from build123d import *

# Parameters (mm, degrees)
F1_DEPTH       = 6.35
F2_R           = 3.81
F3_DEPTH       = 6.35
F5_D           = 2.0574
F5_CSINK_D     = 4.2672
F5_CSINK_ANGLE = 82
F6_D           = 2.032
F6_CSINK_D     = 3.175
F6_CSINK_ANGLE = 82


with BuildPart() as f1:
    # F0 (on Top) → F1 (new body)
    with BuildSketch(Plane.XY):
        with BuildLine():
            ThreePointArc((-6.35, 12.7), (-4.4901280605, 8.2098719395), (0, 6.35))
            Line((0, 6.35), (0, 12.7))
            Line((0, 12.7), (0, 19.05))
            ThreePointArc((0, 19.05), (-4.4901280605, 17.1901280605), (-6.35, 12.7))
        make_face()
        with BuildLine():
            Line((0, 12.7), (0, 6.35))
            ThreePointArc((0, 6.35), (4.4901280605, 8.2098719395), (6.35, 12.7))
            ThreePointArc((6.35, 12.7), (4.4901280605, 17.1901280605), (0, 19.05))
            Line((0, 19.05), (0, 12.7))
        make_face()
        with BuildLine():
            ThreePointArc((6.35, 12.7), (4.4901280605, 8.2098719395), (0, 6.35))
            ThreePointArc((0, 6.35), (-4.4901280605, 8.2098719395), (-6.35, 12.7))
            Line((-6.35, 12.7), (-6.35, 0))
            ThreePointArc((-6.35, 0), (0, -6.35), (6.35, 0))
            Line((6.35, 0), (6.35, 12.7))
        make_face()
        with BuildLine():
            ThreePointArc((0, 19.05), (4.4901280605, 17.1901280605), (6.35, 12.7))
            Line((6.35, 12.7), (6.35, 32.3486101727))
            Line((6.35, 32.3486101727), (5.2643885857, 30.739125063))
            ThreePointArc((5.2643885857, 30.739125063), (2.9811444237, 28.6832827853), (0, 27.94))
            Line((0, 27.94), (0, 19.05))
        make_face()
        with BuildLine():
            Line((-6.35, 34.29), (-6.35, 12.7))
            ThreePointArc((-6.35, 12.7), (-4.4901280605, 17.1901280605), (0, 19.05))
            Line((0, 19.05), (0, 27.94))
            ThreePointArc((0, 27.94), (-4.4901280605, 29.7998719395), (-6.35, 34.29))
        make_face()
        with BuildLine():
            Line((6.35, 34.29), (6.35, 32.3486101727))
            Line((6.35, 32.3486101727), (27.9899881828, 64.4312120116))
            ThreePointArc((27.9899881828, 64.4312120116), (26.2764745341, 73.2464755344), (17.4612110113, 71.5329618857))
            Line((17.4612110113, 71.5329618857), (-5.2643885857, 37.840874937))
            ThreePointArc((-5.2643885857, 37.840874937), (-1.2116371206, 40.5233326149), (3.550874937, 39.5543885857))
            ThreePointArc((3.550874937, 39.5543885857), (5.6067172147, 37.2711444237), (6.35, 34.29))
        make_face()
        with BuildLine():
            Line((5.2643885857, 30.739125063), (6.35, 32.3486101727))
            Line((6.35, 32.3486101727), (6.35, 34.29))
            ThreePointArc((6.35, 34.29), (5.6067172147, 37.2711444237), (3.550874937, 39.5543885857))
            Line((3.550874937, 39.5543885857), (0, 34.29))
            Line((0, 34.29), (0, 27.94))
            ThreePointArc((0, 27.94), (2.9811444237, 28.6832827853), (5.2643885857, 30.739125063))
        make_face()
        with BuildLine():
            ThreePointArc((-5.2643885857, 37.840874937), (-6.0725352004, 36.146560325), (-6.35, 34.29))
            ThreePointArc((-6.35, 34.29), (-4.4901280605, 29.7998719395), (0, 27.94))
            Line((0, 27.94), (0, 34.29))
            Line((0, 34.29), (3.550874937, 39.5543885857))
            ThreePointArc((3.550874937, 39.5543885857), (-1.2116371206, 40.5233326149), (-5.2643885857, 37.840874937))
        make_face()
    extrude(amount=F1_DEPTH)

    # F2 (on face) → F3 (join)
    with BuildSketch(Plane.XY.offset(6.35)):
        with Locations((0, 12.7)):
            Circle(F2_R)
    extrude(amount=F3_DEPTH)

    # F5 (through all)
    with Locations(Plane.XY.offset(12.7)):
        with Locations((0, 12.7)):
            CounterSinkHole(F5_D / 2, F5_CSINK_D / 2, counter_sink_angle=F5_CSINK_ANGLE)

    # F6 (through all)
    with Locations(Plane(origin=(0, 0, 0), x_dir=(1, 0, 0), z_dir=(0, 0, -1))):
        with Locations((0, 0)):
            CounterSinkHole(F6_D / 2, F6_CSINK_D / 2, counter_sink_angle=F6_CSINK_ANGLE)


solid = f1.part
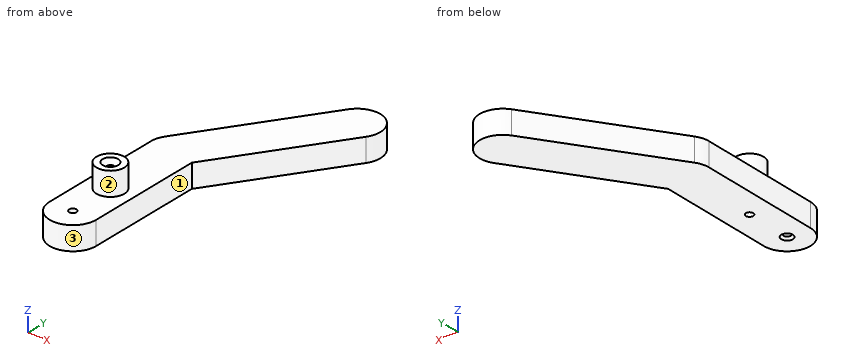
Geometry: final body of the model. Coordinates: model frame, mm. Face numbers are marked on the shaded views. A direction names the side the tool comes from. Give positions to 0.01 mm unless a question says otherwise; leave off trailing zeros. Loops run counter-clockwise (first coordinate to the right, second up) from the corner with the lowest first, then second, coordinate; pieces in that order, holes last. Notation, with made-up numbers: (2, 77) - (44, 77) arc R18 cw to (44, 112) - close; hole circle Ø7 at (0.25, 50.25). An arc over 180 degrees is marked (long way). One line per question, with ' | ' between items. Start each with the question number.
(1) Section query C-C on x = 0. Return loops of the section in (y, z).
(2) Section query A-A on z = 1.75. Return loops of the section in (x, y), then the cut area to 3 significant figures.
(3) Section query D-D on z = 8.5. Return loops of the section in (x, y).
(4) Reachability of the marked faces 1, 2 and 3 from +Z, -Z, +X, -X, +Y, -Y: full face, straight path, thin tool, end or side. Return the list, or none.
(5) Ray query, line 1 (X direction, y = 12.7, z = 6); line 2 (Y direction, x = 0, z = 4.75); line 3 (Z direction, x = 7, y = 37.5). Return the intervals inside material, ascending. Write a range as from..to.
(6) Section query B-B on y = 12.7. Return loops of the section in (x, z), then the cut area to 3 significant figures.
(7) Contact query for flat-ended pins moving along their axis: pin 1 (1.5 mm diameter, centred on x = 11.5, z = 2.5, fed in from +Y); pin 2 (3.5 mm diameter, centred on x = 0, y = 12.7, fed in from +Z); pin 3 (10.5 mm diameter, centred on x = 15, y = 38.5, fed in from +Z). Output: stop coordinate, or through.
The answers:
1) outline: (-6.35, 0) - (-1.59, 0) - (-1.02, 0.66) - (-1.02, 6.35) - (-6.35, 6.35) - close; (1.02, 0.66) - (1.59, 0) - (11.67, 0) - (11.67, 11.43) - (10.57, 12.7) - (8.89, 12.7) - (8.89, 6.35) - (1.02, 6.35) - close; (13.73, 0) - (45.65, 0) - (45.65, 6.35) - (16.51, 6.35) - (16.51, 12.7) - (14.83, 12.7) - (13.73, 11.43) - close
2) outline: (-6.35, 0) arc R6.35 ccw to (6.35, 0) - (6.35, 32.35) - (27.99, 64.43) arc R6.35 ccw to (17.46, 71.53) - (-5.26, 37.84) arc R6.35 ccw to (-6.35, 34.29) - close; hole circle Ø2.06 at (0, 12.7); hole circle Ø2.03 at (0, 0) | area: 1,070 mm2
3) outline: circle Ø7.62 at (0, 12.7); hole circle Ø2.06 at (0, 12.7)
4) face 1: +Z, -Z, +X, -Y | face 2: +Z | face 3: +Z, -Z, -Y
5) line 1: -6.35..-1.03, 1.03..6.35 | line 2: -6.35..-1.02, 1.02..11.67, 13.73..45.65 | line 3: 0..6.35
6) outline: (-6.35, 0) - (-1.03, 0) - (-1.03, 11.43) - (-2.13, 12.7) - (-3.81, 12.7) - (-3.81, 6.35) - (-6.35, 6.35) - close; (1.03, 0) - (6.35, 0) - (6.35, 6.35) - (3.81, 6.35) - (3.81, 12.7) - (2.13, 12.7) - (1.03, 11.43) - close | area: 101 mm2
7) pin 1: y = 63.81 | pin 2: z = 12.26 | pin 3: z = 6.35
